```python
from build123d import *

# Parameters (mm, degrees)
SKETCH1_W                                     = 144
SKETCH1_H                                     = 270
SKETCH1_R                                     = 17
BASE_FLANGE1_DEPTH                            = 14
CBORE_FOR_M8_HEX_SOCKET_HEAD_CAP_SCR_2_COUNT  = 2
CBORE_FOR_M8_HEX_SOCKET_HEAD_CAP_SCR_2_PITCH  = 30
CBORE_FOR_M8_HEX_SOCKET_HEAD_CAP_SCR_3_COUNT  = 2
CBORE_FOR_M8_HEX_SOCKET_HEAD_CAP_SCR_3_PITCH  = 42.426406871
CBORE_FOR_M8_HEX_SOCKET_HEAD_CAP_SCR_4_COUNT  = 2
CBORE_FOR_M8_HEX_SOCKET_HEAD_CAP_SCR_4_PITCH  = 30
CBORE_FOR_M8_HEX_SOCKET_HEAD_CAP_SCR_5_COUNT  = 2
CBORE_FOR_M8_HEX_SOCKET_HEAD_CAP_SCR_5_PITCH  = 241.867732449
CBORE_FOR_M8_HEX_SOCKET_HEAD_CAP_SCR_6_COUNT  = 2
CBORE_FOR_M8_HEX_SOCKET_HEAD_CAP_SCR_6_PITCH  = 240
CBORE_FOR_M8_HEX_SOCKET_HEAD_CAP_SCR_7_COUNT  = 2
CBORE_FOR_M8_HEX_SOCKET_HEAD_CAP_SCR_7_PITCH  = 212.132034356
CBORE_FOR_M8_HEX_SOCKET_HEAD_CAP_SCR_8_COUNT  = 2
CBORE_FOR_M8_HEX_SOCKET_HEAD_CAP_SCR_8_PITCH  = 210
M4_TAPPED_HOLE1_D                             = 3.3
M4_TAPPED_HOLE1_CSINK_D                       = 4.05
M4_TAPPED_HOLE1_CSINK_ANGLE                   = 90
M5_CLEARANCE_HOLE1_AT_2_COUNT                 = 2
M5_CLEARANCE_HOLE1_AT_2_PITCH                 = 47.100382695
M5_CLEARANCE_HOLE1_AT_3_COUNT                 = 2
M5_CLEARANCE_HOLE1_AT_3_PITCH                 = 66.61
M5_CLEARANCE_HOLE1_AT_4_COUNT                 = 2
M5_CLEARANCE_HOLE1_AT_4_PITCH                 = 47.100382695
CBORE_FOR_M6_HEX_SOCKET_HEAD_CAP_SCR_2_COUNT  = 2
CBORE_FOR_M6_HEX_SOCKET_HEAD_CAP_SCR_2_PITCH  = 114
CRVPATTERN1_COUNT                             = 2
CRVPATTERN1_PITCH                             = 70
M4_TAPPED_HOLE2_AT_2_COUNT                    = 2
M4_TAPPED_HOLE2_AT_2_PITCH                    = 142.214626533
M4_TAPPED_HOLE2_AT_3_COUNT                    = 2
M4_TAPPED_HOLE2_AT_3_PITCH                    = 254
M4_TAPPED_HOLE2_AT_4_COUNT                    = 2
M4_TAPPED_HOLE2_AT_4_PITCH                    = 142.214626533
CBORE_FOR_M8_HEX_SOCKET_HEAD_CAP_SCR_9_COUNT  = 2
CBORE_FOR_M8_HEX_SOCKET_HEAD_CAP_SCR_9_PITCH  = 30
CBORE_FOR_M8_HEX_SOCKET_HEAD_CAP_SCR_10_COUNT = 2
CBORE_FOR_M8_HEX_SOCKET_HEAD_CAP_SCR_10_PITCH = 210
CBORE_FOR_M8_HEX_SOCKET_HEAD_CAP_SCR_11_COUNT = 2
CBORE_FOR_M8_HEX_SOCKET_HEAD_CAP_SCR_11_PITCH = 240
CBORE_FOR_M8_HEX_SOCKET_HEAD_CAP_SCR_12_COUNT = 2
CBORE_FOR_M8_HEX_SOCKET_HEAD_CAP_SCR_12_PITCH = 212.132034356
CBORE_FOR_M8_HEX_SOCKET_HEAD_CAP_SCR_13_COUNT = 2
CBORE_FOR_M8_HEX_SOCKET_HEAD_CAP_SCR_13_PITCH = 241.867732449
FILLET1_R                                     = 3
CHAMFER1_SIZE                                 = 0.8


# Sheet-metal steps are written as plain solids
with BuildPart() as part:
    # Sketch1 → Base-Flange1 (new body)
    with BuildSketch(Plane.XY):
        with Locations((-72, -135)):
            Rectangle(SKETCH1_W, SKETCH1_H)
        with Locations(Location((-70, -90, 0), (0, 0, 180))):
            Circle(SKETCH1_R, mode=Mode.SUBTRACT)
    extrude(amount=-BASE_FLANGE1_DEPTH)

    # Sketch7 → CBORE for M8 Hex Socket Head Cap Screw1 (revolve, cut)
    with BuildSketch(Plane(origin=(-45, -15, 0), x_dir=(0, -1, 0), z_dir=(1, 0, 0))):
        Polygon((0, 0), (0, 14), (4.75, 14), (4.25, 13.5), (4.25, 9), (7, 9), (7, 0.25), (7.25, 0), align=None)
    cbore_for_m8_hex_socket_head_cap_screw1 = revolve(axis=Axis((-45, -15, 6.35), (0, 0, -1)), mode=Mode.SUBTRACT)

    # CBORE for M8 Hex Socket Head Cap Scr 2: CBORE for M8 Hex Socket Head Cap Screw1 ×2
    with Locations(*[(i * CBORE_FOR_M8_HEX_SOCKET_HEAD_CAP_SCR_2_PITCH, 0, 0) for i in range(1, CBORE_FOR_M8_HEX_SOCKET_HEAD_CAP_SCR_2_COUNT)]):
        add(cbore_for_m8_hex_socket_head_cap_screw1, mode=Mode.SUBTRACT)

    # CBORE for M8 Hex Socket Head Cap Scr 3: CBORE for M8 Hex Socket Head Cap Screw1 ×2
    with Locations(*[Vector(0.7071067811865476, -0.7071067811865475, 0) * (i * CBORE_FOR_M8_HEX_SOCKET_HEAD_CAP_SCR_3_PITCH) for i in range(1, CBORE_FOR_M8_HEX_SOCKET_HEAD_CAP_SCR_3_COUNT)]):
        add(cbore_for_m8_hex_socket_head_cap_screw1, mode=Mode.SUBTRACT)

    # CBORE for M8 Hex Socket Head Cap Scr 4: CBORE for M8 Hex Socket Head Cap Screw1 ×2
    with Locations(*[(0, -i * CBORE_FOR_M8_HEX_SOCKET_HEAD_CAP_SCR_4_PITCH, 0) for i in range(1, CBORE_FOR_M8_HEX_SOCKET_HEAD_CAP_SCR_4_COUNT)]):
        add(cbore_for_m8_hex_socket_head_cap_screw1, mode=Mode.SUBTRACT)

    # CBORE for M8 Hex Socket Head Cap Scr 5: CBORE for M8 Hex Socket Head Cap Screw1 ×2
    with Locations(*[Vector(0.12403473458920848, -0.9922778767136676, 0) * (i * CBORE_FOR_M8_HEX_SOCKET_HEAD_CAP_SCR_5_PITCH) for i in range(1, CBORE_FOR_M8_HEX_SOCKET_HEAD_CAP_SCR_5_COUNT)]):
        add(cbore_for_m8_hex_socket_head_cap_screw1, mode=Mode.SUBTRACT)

    # CBORE for M8 Hex Socket Head Cap Scr 6: CBORE for M8 Hex Socket Head Cap Screw1 ×2
    with Locations(*[(0, -i * CBORE_FOR_M8_HEX_SOCKET_HEAD_CAP_SCR_6_PITCH, 0) for i in range(1, CBORE_FOR_M8_HEX_SOCKET_HEAD_CAP_SCR_6_COUNT)]):
        add(cbore_for_m8_hex_socket_head_cap_screw1, mode=Mode.SUBTRACT)

    # CBORE for M8 Hex Socket Head Cap Scr 7: CBORE for M8 Hex Socket Head Cap Screw1 ×2
    with Locations(*[Vector(0.1414213562373096, -0.9899494936611666, 0) * (i * CBORE_FOR_M8_HEX_SOCKET_HEAD_CAP_SCR_7_PITCH) for i in range(1, CBORE_FOR_M8_HEX_SOCKET_HEAD_CAP_SCR_7_COUNT)]):
        add(cbore_for_m8_hex_socket_head_cap_screw1, mode=Mode.SUBTRACT)

    # CBORE for M8 Hex Socket Head Cap Scr 8: CBORE for M8 Hex Socket Head Cap Screw1 ×2
    with Locations(*[(0, -i * CBORE_FOR_M8_HEX_SOCKET_HEAD_CAP_SCR_8_PITCH, 0) for i in range(1, CBORE_FOR_M8_HEX_SOCKET_HEAD_CAP_SCR_8_COUNT)]):
        add(cbore_for_m8_hex_socket_head_cap_screw1, mode=Mode.SUBTRACT)

    # M4 Tapped Hole1 (through all)
    with Locations(Plane.XY):
        with Locations((-91, -90), (-70, -69), (-49, -90), (-70, -111)):
            CounterSinkHole(M4_TAPPED_HOLE1_D / 2, M4_TAPPED_HOLE1_CSINK_D / 2, counter_sink_angle=M4_TAPPED_HOLE1_CSINK_ANGLE)

    # Sketch16 → M5 Clearance Hole1 (revolve, cut)
    with BuildSketch(Plane(origin=(-93.550191347, -113.550191347, 0), x_dir=(0, -1, 0), z_dir=(1, 0, 0))):
        Polygon((0, 0), (0, 14), (3, 14), (2.75, 13.75), (2.75, 0.25), (3, 0), align=None)
    m5_clearance_hole1 = revolve(axis=Axis((-93.550191347, -113.550191347, 6.35), (0, 0, -1)), mode=Mode.SUBTRACT)

    # M5 Clearance Hole1 at 2: M5 Clearance Hole1 ×2
    with Locations(*[(0, i * M5_CLEARANCE_HOLE1_AT_2_PITCH, 0) for i in range(1, M5_CLEARANCE_HOLE1_AT_2_COUNT)]):
        add(m5_clearance_hole1, mode=Mode.SUBTRACT)

    # M5 Clearance Hole1 at 3: M5 Clearance Hole1 ×2
    with Locations(*[Vector(0.707106781186551, 0.707106781186544, 0) * (i * M5_CLEARANCE_HOLE1_AT_3_PITCH) for i in range(1, M5_CLEARANCE_HOLE1_AT_3_COUNT)]):
        add(m5_clearance_hole1, mode=Mode.SUBTRACT)

    # M5 Clearance Hole1 at 4: M5 Clearance Hole1 ×2
    with Locations(*[(i * M5_CLEARANCE_HOLE1_AT_4_PITCH, 0, 0) for i in range(1, M5_CLEARANCE_HOLE1_AT_4_COUNT)]):
        add(m5_clearance_hole1, mode=Mode.SUBTRACT)

    # Sketch20 → CBORE for M6 Hex Socket Head Cap Screw1 (revolve, cut)
    with BuildSketch(Plane(origin=(-129, -100, 0), x_dir=(0, -1, 0), z_dir=(1, 0, 0))):
        Polygon((0, 0), (0, 14), (3.5, 14), (3.25, 13.75), (3.25, 8), (5.5, 8), (5.5, 0.25), (5.75, 0), align=None)
    cbore_for_m6_hex_socket_head_cap_screw1 = revolve(axis=Axis((-129, -100, 6.35), (0, 0, -1)), mode=Mode.SUBTRACT)

    # CBORE for M6 Hex Socket Head Cap Scr 2: CBORE for M6 Hex Socket Head Cap Screw1 ×2
    with Locations(*[(i * CBORE_FOR_M6_HEX_SOCKET_HEAD_CAP_SCR_2_PITCH, 0, 0) for i in range(1, CBORE_FOR_M6_HEX_SOCKET_HEAD_CAP_SCR_2_COUNT)]):
        add(cbore_for_m6_hex_socket_head_cap_screw1, mode=Mode.SUBTRACT)

    # CrvPattern1: CBORE for M6 Hex Socket Head Cap Screw1 ×2
    with Locations(*[(0, -i * CRVPATTERN1_PITCH, 0) for i in range(1, CRVPATTERN1_COUNT)]):
        add(cbore_for_m6_hex_socket_head_cap_screw1, mode=Mode.SUBTRACT)

    # CrvPattern1 copy 1 sketch → CrvPattern1 copy 1 (revolve, cut)
    with BuildSketch(Plane(origin=(-15, -170, 0), x_dir=(0, -1, 0), z_dir=(1, 0, 0))):
        Polygon((0, 0), (0, 14), (3.5, 14), (3.25, 13.75), (3.25, 8), (5.5, 8), (5.5, 0.25), (5.75, 0), align=None)
    revolve(axis=Axis((-15, -170, 6.35), (0, 0, -1)), mode=Mode.SUBTRACT)

    # Sketch26 → M4 Tapped Hole2 (revolve, cut)
    with BuildSketch(Plane(origin=(-72, -8, 0), x_dir=(0, -1, 0), z_dir=(1, 0, 0))):
        Polygon((0, 0), (0, 14), (2.025, 14), (1.65, 13.625), (1.65, 0), align=None)
    m4_tapped_hole2 = revolve(axis=Axis((-72, -8, 6.35), (0, 0, -1)), mode=Mode.SUBTRACT)

    # M4 Tapped Hole2 at 2: M4 Tapped Hole2 ×2
    with Locations(*[Vector(-0.45002403451816303, -0.8930164434969803, 0) * (i * M4_TAPPED_HOLE2_AT_2_PITCH) for i in range(1, M4_TAPPED_HOLE2_AT_2_COUNT)]):
        add(m4_tapped_hole2, mode=Mode.SUBTRACT)

    # M4 Tapped Hole2 at 3: M4 Tapped Hole2 ×2
    with Locations(*[(0, -i * M4_TAPPED_HOLE2_AT_3_PITCH, 0) for i in range(1, M4_TAPPED_HOLE2_AT_3_COUNT)]):
        add(m4_tapped_hole2, mode=Mode.SUBTRACT)

    # M4 Tapped Hole2 at 4: M4 Tapped Hole2 ×2
    with Locations(*[Vector(0.4500240345181632, -0.8930164434969802, 0) * (i * M4_TAPPED_HOLE2_AT_4_PITCH) for i in range(1, M4_TAPPED_HOLE2_AT_4_COUNT)]):
        add(m4_tapped_hole2, mode=Mode.SUBTRACT)

    # Sketch28 → CBORE for M8 Hex Socket Head Cap Screw2 (revolve, cut)
    with BuildSketch(Plane(origin=(-129, -15, 0), x_dir=(0, -1, 0), z_dir=(1, 0, 0))):
        Polygon((0, 0), (0, 14), (4.75, 14), (4.25, 13.5), (4.25, 9), (7, 9), (7, 0.75), (7.75, 0), align=None)
    cbore_for_m8_hex_socket_head_cap_screw2 = revolve(axis=Axis((-129, -15, 6.35), (0, 0, -1)), mode=Mode.SUBTRACT)

    # CBORE for M8 Hex Socket Head Cap Scr 9: CBORE for M8 Hex Socket Head Cap Screw2 ×2
    with Locations(*[(0, -i * CBORE_FOR_M8_HEX_SOCKET_HEAD_CAP_SCR_9_PITCH, 0) for i in range(1, CBORE_FOR_M8_HEX_SOCKET_HEAD_CAP_SCR_9_COUNT)]):
        add(cbore_for_m8_hex_socket_head_cap_screw2, mode=Mode.SUBTRACT)

    # CBORE for M8 Hex Socket Head Cap Scr 10: CBORE for M8 Hex Socket Head Cap Screw2 ×2
    with Locations(*[(0, -i * CBORE_FOR_M8_HEX_SOCKET_HEAD_CAP_SCR_10_PITCH, 0) for i in range(1, CBORE_FOR_M8_HEX_SOCKET_HEAD_CAP_SCR_10_COUNT)]):
        add(cbore_for_m8_hex_socket_head_cap_screw2, mode=Mode.SUBTRACT)

    # CBORE for M8 Hex Socket Head Cap Scr 11: CBORE for M8 Hex Socket Head Cap Screw2 ×2
    with Locations(*[(0, -i * CBORE_FOR_M8_HEX_SOCKET_HEAD_CAP_SCR_11_PITCH, 0) for i in range(1, CBORE_FOR_M8_HEX_SOCKET_HEAD_CAP_SCR_11_COUNT)]):
        add(cbore_for_m8_hex_socket_head_cap_screw2, mode=Mode.SUBTRACT)

    # CBORE for M8 Hex Socket Head Cap Scr 12: CBORE for M8 Hex Socket Head Cap Screw2 ×2
    with Locations(*[Vector(0.14142135623730956, -0.9899494936611666, 0) * (i * CBORE_FOR_M8_HEX_SOCKET_HEAD_CAP_SCR_12_PITCH) for i in range(1, CBORE_FOR_M8_HEX_SOCKET_HEAD_CAP_SCR_12_COUNT)]):
        add(cbore_for_m8_hex_socket_head_cap_screw2, mode=Mode.SUBTRACT)

    # CBORE for M8 Hex Socket Head Cap Scr 13: CBORE for M8 Hex Socket Head Cap Screw2 ×2
    with Locations(*[Vector(0.12403473458920847, -0.9922778767136677, 0) * (i * CBORE_FOR_M8_HEX_SOCKET_HEAD_CAP_SCR_13_PITCH) for i in range(1, CBORE_FOR_M8_HEX_SOCKET_HEAD_CAP_SCR_13_COUNT)]):
        add(cbore_for_m8_hex_socket_head_cap_screw2, mode=Mode.SUBTRACT)

    # Fillet1
    fillet1_edges = [part.edges().sort_by_distance(p)[0] for p in [
        (0, 0, -7),
        (0, -270, -7),
        (-144, -270, -7),
        (-144, 0, -7),
    ]]
    fillet(fillet1_edges, radius=FILLET1_R)

    # Chamfer1
    chamfer1_edges = [part.edges().sort_by_distance(p)[0] for p in [
        (-53, -90, -14),
        (-53, -90, 0),
        (-72, -270, 0),
        (-72, -270, -14),
        (-72, 0, 0),
        (-144, -135, 0),
        (0, -135, 0),
        (-143.121320344, -0.878679656, 0),
        (-143.121320344, -269.121320344, 0),
        (-0.878679656, -0.878679656, 0),
        (-0.878679656, -269.121320344, 0),
        (0, -135, -14),
        (-72, 0, -14),
        (-144, -135, -14),
        (-143.121320344, -0.878679656, -14),
        (-143.121320344, -269.121320344, -14),
        (-0.878679656, -0.878679656, -14),
        (-0.878679656, -269.121320344, -14),
    ]]
    chamfer(chamfer1_edges, length=CHAMFER1_SIZE)


solid = part.part
```
Build history of the part. All positions in model axes, mm. A direction names the side the tool comes from. Give positions to 0.01 mm unless a question says otherwise; leave off trailing zeros.
Item 1: Drill centre lines: line 1 (X direction, y = -255, z = -5.25); line 2 (X direction, y = -170, z = -4.75); line 3 (Y direction, x = -73.5, z = -12.75). Where is each one in solid material? Low to high.
Answers follow:
line 1: x = -144 to -136, -122 to -106, -92 to -52, -38 to -22, -8 to 0
line 2: x = -144 to -134.5, -123.5 to -20.5, -9.5 to 0
line 3: y = -270 to -262.69, -261.31 to -106.64, -73.36 to -8.69, -7.31 to 0
Item 2: Pull direction X, two halves, no side cores. Call faces 3 (the face through (0, -137, -7)), 4 (the face through (-129, -96, -8)), 5 (the face through (-15.242, -164.505, -4.071)): released by +X, released by -X, zero draft, split by the parting line, or undercut.
Answers follow:
face 3: released by +X
face 4: undercut
face 5: undercut
Item 3: Flat gauge pin, fed straight in: pin 1 (7 mm diameter, centred on x = -14, y = -256, fed in from +Z). Where does the tip first touch, or does it go through?
Answers follow:
pin 1: stops at z = -9
Item 4: Which spindle directions (+Z, -Z, +X, -X, +Y, -Y) get a long thin tool onto all of the face, cutting with end or side? Do faces 1 (the face through (-96.277, -66.092, -6.906)), 2 (the face through (-15, -38, -5)). Say none if no direction does.
Answers follow:
face 1: +Z, -Z
face 2: +Z
Item 5: Slice it at A-A, the plane y = -255. Give the number of separate pieces and of enclosed holes in the cut face, and give its area (3 significant figures).
Answers follow:
separate pieces: 5
enclosed holes: 0
area: 1,340 mm2
